Part model, mm, in its own coordinate system. Face numbers are marked on the shaded views. A direction names the side the tool comes from. Give positions to 0.01 mm unless a question says otherwise; leave off trailing zeros. Order: outer loops, then holes, each group sorted by start corner. A loop starts at its lowest first (then second) coordinate and runs counter-clockwise, first axis right, second up. Notation, with made-up numbers: M -39.75,-10.75 L -32.75,-10.75 A9 ccw -32.75,-3.75 Z; hole C -23.75,84.5 d2. An arc over 180 degrees is marked long. One line per question, with ' | ' between items.
```python
from build123d import *

# Parameters (mm, degrees)
ESBO_O2_R                  = 5
RESSALTO_EXTRUS_O1_DEPTH   = 20
ESBO_O3_R                  = 4
RESSALTO_EXTRUS_O2_DEPTH   = 20
ESBO_O4_R                  = 2
RESSALTO_EXTRUS_O3_DEPTH   = 10
CHANFRO1_SIZE              = 0.625
CHANFRO2_SIZE              = 0.35
CORTE_EXTRUS_O2_DEPTH      = 31.822070015
CORTE_EXTRUS_O2_DEPTH_BACK = 31.822070015
ESBO_O6_W                  = 1
ESBO_O6_H                  = 5


with BuildPart() as part:
    # Esboço2 → Ressalto-extrusão1 (new body)
    with BuildSketch(Plane.XY):
        Circle(ESBO_O2_R)
    extrude(amount=-RESSALTO_EXTRUS_O1_DEPTH)

    # Esboço3 → Ressalto-extrusão2 (add)
    with BuildSketch(Plane.XY):
        Circle(ESBO_O3_R)
    extrude(amount=RESSALTO_EXTRUS_O2_DEPTH)

    # Esboço4 → Ressalto-extrusão3 (add)
    with BuildSketch(Plane(origin=(0, 0, -20), x_dir=(-1, 0, 0), z_dir=(0, 0, -1))):
        Circle(ESBO_O4_R)
    extrude(amount=RESSALTO_EXTRUS_O3_DEPTH)

    # Chanfro1
    chanfro1_edges = [part.edges().sort_by_distance(p)[0] for p in [
        (-4, 0, 20),
    ]]
    chamfer(chanfro1_edges, length=CHANFRO1_SIZE)

    # Chanfro2
    chanfro2_edges = [part.edges().sort_by_distance(p)[0] for p in [
        (2, 0, -30),
    ]]
    chamfer(chanfro2_edges, length=CHANFRO2_SIZE)

    # Esboço6 → Corte-extrusão2 (cut, two sides: drawn at the far end of the back side and taken through both)
    with BuildSketch(Plane(origin=(0, 0, 0), x_dir=(1, 0, 0), z_dir=(0, 1, 0)).offset(-CORTE_EXTRUS_O2_DEPTH_BACK)):
        with Locations((-4.5, 17.5)):
            Rectangle(ESBO_O6_W, ESBO_O6_H)
        with Locations((-4.5, 2.5)):
            Rectangle(ESBO_O6_W, ESBO_O6_H)
        with Locations((4.5, 17.5)):
            Rectangle(ESBO_O6_W, ESBO_O6_H)
        with Locations((4.5, 2.5)):
            Rectangle(ESBO_O6_W, ESBO_O6_H)
    extrude(amount=CORTE_EXTRUS_O2_DEPTH + CORTE_EXTRUS_O2_DEPTH_BACK, mode=Mode.SUBTRACT)


solid = part.part
```
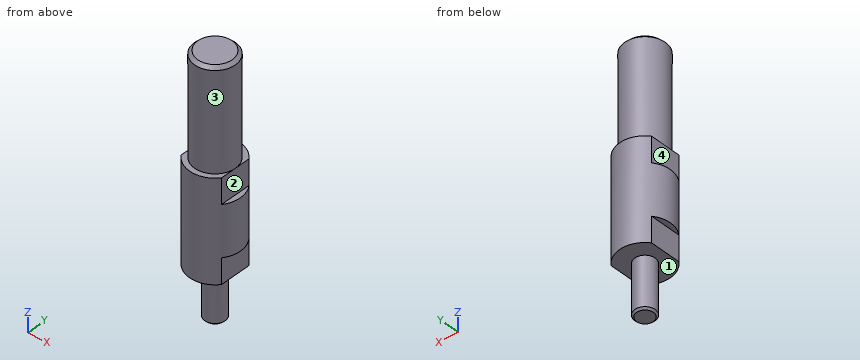
1. Drop flat-ended pins along their axis: pin 1 (1.5 mm diameter, centred on y = -0.5, z = -17.5, fed in from +X); pin 2 (1.1 mm diameter, centred on x = -4.5, y = 0, fed in from -Z); pin 3 (2.5 mm diameter, centred on y = -0.5, z = -3, fed in from -X). Give the stop position or say it passes through.
Worked out:
pin 1: stops at x = 4 | pin 2: stops at z = -20 | pin 3: stops at x = -4
2. Slice it at C-C on z = 16.5. Give the cut face in (x, y).
Worked out:
outline: C 0,0 d8
3. Probe L1, parallel to X at y = 0.25, z = 2; L2, parallel to Y at x = 0.25, z = -19.5; L3, parallel to Z at x = 0, y = 3.25. List the from-to ranges inside material, lowest first. Write a range as from..to.
Worked out:
L1: x = -3.99..3.99 | L2: y = -4.99..4.99 | L3: z = -20..20
4. Slice it at A-A on x = 0. Give the cut face in (y, z) (3 decimals).
Worked out:
outline: M -5,-20 L -2,-20 L -2,-29.65 L -1.65,-30 L 1.65,-30 L 2,-29.65 L 2,-20 L 5,-20 L 5,0 L 4,0 L 4,19.375 L 3.375,20 L -3.375,20 L -4,19.375 L -4,0 L -5,0 Z
5. Tool access for the marked faces 1, 2, 3 and 4: list every direction of +Z, -Z, +X, -X, +Y, -Y with a clear straight run to the whole face (end or side of a thin tool).
Worked out:
face 1: -Z | face 2: +Z, +X, +Y, -Y | face 3: +Z | face 4: +Z, -X, +Y, -Y
6. Slice it at B-B on z = -23.5. Give the cut face in (x, y).
Worked out:
outline: C 0,0 d4
